Part print with two shaded views. Sizes in mm from the minimum x, y, z corner. A direction names the side the tool comes from. Round coordinates to 2 decimals unless told otherwise and drop trailing zeros. Order: outer loops, then holes, each group sorted by start corner. A loop starts at its lowest first (then second) coordinate and runs counter-clockwise, first axis right, second up. Notation, with made-up numbers: M -33.5,-1.5 L -18.5,-1.5 A25 ccw -18.5,12.5 Z; hole C 8.25,42.5 d11. An arc over 180 degrees is marked long. Put each result on its own line as item: value.
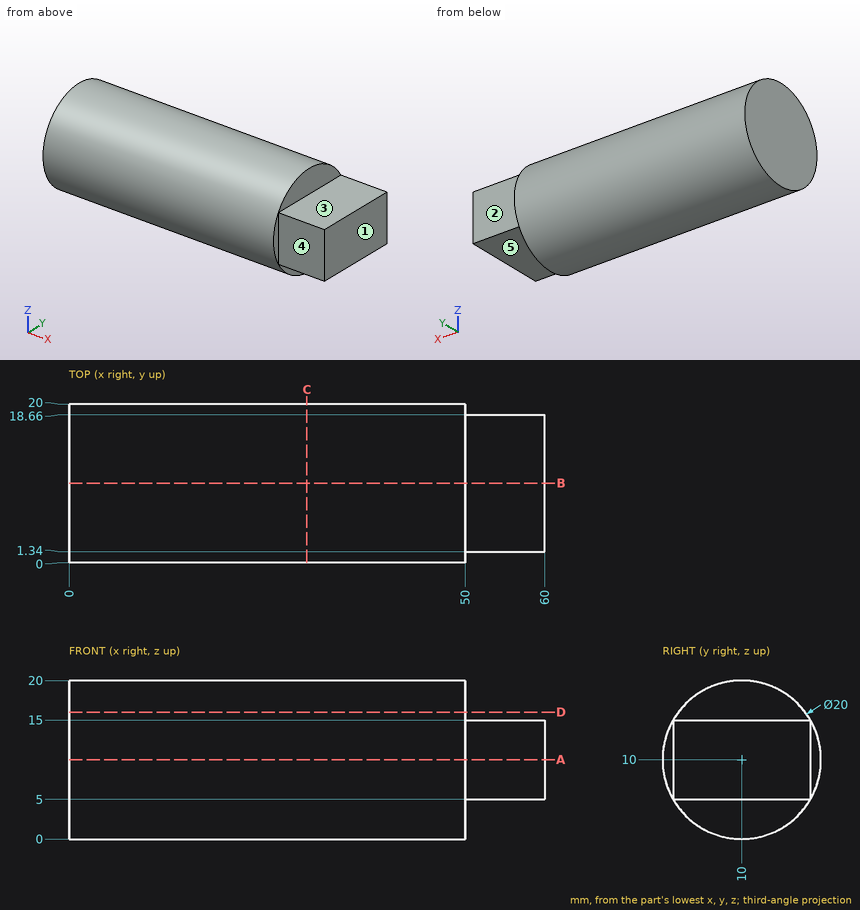
Item 1: Tool access for the marked faces 1, 2, 3, 4 and 5: list every direction of +Z, -Z, +X, -X, +Y, -Y with a clear straight run to the whole face (end or side of a thin tool).
Answers below:
face 1: +Z, -Z, +X, +Y, -Y
face 2: +Z, -Z, +X, +Y
face 3: +Z, +X, +Y, -Y
face 4: +Z, -Z, +X, -Y
face 5: -Z, +X, +Y, -Y
Item 2: Band-saw the part on B-B on y = 10. Give the cut face in (x, z), and give its area (3 significant figures).
Answers below:
outline: M 0,0 L 50,0 L 50,5 L 60,5 L 60,15 L 50,15 L 50,20 L 0,20 Z
area: 1,100 mm²
Item 3: Band-saw the part on A-A on z = 10. Give the cut face in (x, y), and give its area (3 significant figures).
Answers below:
outline: M 0,0 L 50,0 L 50,1.34 L 60,1.34 L 60,18.66 L 50,18.66 L 50,20 L 0,20 Z
area: 1,170 mm²
Item 4: Probe line 1 along X through (y, z) = (15.75, 3.5); line 2 along Y through (x, z) = (52, 12); line 3 along Z through (x, y) = (41, 10.5). List the from-to ranges inside material, lowest first. Write a range as [from, to].
Answers below:
line 1: [0, 50]
line 2: [1.34, 18.66]
line 3: [0.01, 19.99]
Item 5: Band-saw the part on C-C on x = 30. Give the cut face in (y, z).
Answers below:
outline: C 10,10 d20
Item 6: Pin check, flat tips, straight feed: P1, Ø3, axis at x = 55, z = 9.5, coming from the +Y side; P2, Ø1.1, axis at y = 0.5, z = 12, coming from the +X side; P3, Ø5, axis at x = 35, z = 14.5, coming from the -Y side. Stop position of each tip, or through.
Answers below:
P1: y = 18.66
P2: x = 50
P3: y = 0.2
Item 7: Band-saw the part on D-D on z = 16. Give the cut face in (x, y), and give its area (3 significant figures).
Answers below:
outline: M 0,2 L 50,2 L 50,18 L 0,18 Z
area: 800 mm²
